from build123d import *

# Parameters (mm, degrees)
F1_DEPTH = 10
F2_R     = 2
F3_R     = 4.4
F4_R     = 4
F5_R     = 6.2


with BuildPart() as f1:
    # F0 (on Top) → F1 (new body)
    with BuildSketch(Plane.XY):
        Polygon((6.78689, 27.703254), (6.78689, 2.703254), (9.18689, 2.703254), (9.18689, 30.103254), (-16.61311, 30.103254), (-16.61311, -19.896746), (-24.81311, -19.896746), (-24.81311, -7.296746), (-27.21311, -7.296746), (-27.21311, -22.296746), (-14.21311, -22.296746), (-14.21311, 27.703254), align=None)
    extrude(amount=F1_DEPTH)

    # F2
    f2_edges = [f1.edges().sort_by_distance(p)[0] for p in [
        (-14.21311, 27.703254, 5),
        (6.78689, 27.703254, 5),
    ]]
    fillet(f2_edges, radius=F2_R)

    # F3
    f3_edges = [f1.edges().sort_by_distance(p)[0] for p in [
        (-16.61311, 30.103254, 5),
        (9.18689, 30.103254, 5),
    ]]
    fillet(f3_edges, radius=F3_R)

    # F4
    f4_edges = [f1.edges().sort_by_distance(p)[0] for p in [
        (-24.81311, -19.896746, 5),
        (-16.61311, -19.896746, 5),
    ]]
    fillet(f4_edges, radius=F4_R)

    # F5
    f5_edges = [f1.edges().sort_by_distance(p)[0] for p in [
        (-27.21311, -22.296746, 5),
        (-14.21311, -22.296746, 5),
    ]]
    fillet(f5_edges, radius=F5_R)


solid = f1.part
Build history of the part. All positions in model axes, mm. A direction names the side the tool comes from. Round coordinates to 2 decimals unless told otherwise and drop trailing zeros. Loops run counter-clockwise (first coordinate to the right, second up) from the corner with the lowest first, then second, coordinate; pieces in that order, holes last. Notation, with made-up numbers: (10.25, -8) -> (44.25, -8) arc R20 ccw to (44.25, 7) -> close; hole circle Ø7 at (44.25, -12.5). An arc over 180 degrees is marked (long way). Use CSV: the item, a comma, the result in double quotes. Start each with the question number.
Q1. Saw through at D-D on y = 0. Give the cut face in (x, z), and give its area (3 significant figures).
Q2. Saw through at B-B on z = 4.5. Give the cut face in (x, y).
Q3. Saw through at A-A on y = 24.5. Give the cut face in (x, z), and give its area (3 significant figures).
Q4. Mould opens along X. For faces 4 (the face through (9.187, 14, 5)), 5 (the face through (-14.213, 5, 5)), 6 (the face through (-26, -7.297, 5)) say: +X half, -X half, draft (parallel to the pull), parting line (faces both ways), or undercut.
Q5. Saw through at C-C on x = -4.5. Give the cut face in (y, z), and give its area (3 significant figures).
Q6. Flat gauge pins, fed straight in: pin 1 Ø2.5 at (y, z) = (-13, 6.5) entering from +X; pin 2 Ø2.5 at (x, z) = (-26.5, 4.5) entering from +Y; pin 3 Ø3 at (y, z) = (-2.5, 6) entering from -X; pin 4 Ø1.5 at (x, y) = (-12.5, -3.5) entering from -Z. Where does each tip first touch, or does it go through?
Q7. Drill centre lines: L1, parallel to X at y = 21, z = 4; L2, parallel to X at y = -15, z = 8.75; L3, parallel to Y at x = -5.5, z = 1. Where is each one in solid material? Low to high.
Q8. Which spindle directions (+Z, -Z, +X, -X, +Y, -Y) get a long thin tool onto all of the face, cutting with end or side? Do faces 1 (the face through (-24.813, -12, 5)), 2 (the face through (-13.643, 27.102, 5.07)), 3 (the face through (8, 2.703, 5)). Say none if no direction does.
Solutions:
1,outline,"(-16.61, 0) -> (-14.21, 0) -> (-14.21, 10) -> (-16.61, 10) -> close"
1,area,"24.0 mm^2"
2,outline,"(-27.21, -16.1) arc R6.2 ccw to (-21.01, -22.3) -> (-20.41, -22.3) arc R6.2 ccw to (-14.21, -16.1) -> (-14.21, 25.7) arc R2 cw to (-12.21, 27.7) -> (4.79, 27.7) arc R2 cw to (6.79, 25.7) -> (6.79, 2.7) -> (9.19, 2.7) -> (9.19, 25.7) arc R4.4 ccw to (4.79, 30.1) -> (-12.21, 30.1) arc R4.4 ccw to (-16.61, 25.7) -> (-16.61, -15.9) arc R4 cw to (-20.61, -19.9) -> (-20.81, -19.9) arc R4 cw to (-24.81, -15.9) -> (-24.81, -7.3) -> (-27.21, -7.3) -> close"
3,outline,"(-16.61, 0) -> (-14.21, 0) -> (-14.21, 10) -> (-16.61, 10) -> close; (6.79, 0) -> (9.19, 0) -> (9.19, 10) -> (6.79, 10) -> close"
3,area,"48.0 mm^2"
4,face 4,"+X half"
4,face 5,"undercut"
4,face 6,"draft"
5,outline,"(27.7, 0) -> (30.1, 0) -> (30.1, 10) -> (27.7, 10) -> close"
5,area,"24.0 mm^2"
6,pin 1,"stops at x = -14.21"
6,pin 2,"stops at y = -7.3"
6,pin 3,"stops at x = -16.61"
6,pin 4,"passes through"
7,L1,"x = -16.61 to -14.21, 6.79 to 9.19"
7,L2,"x = -27.21 to -24.81, -16.61 to -14.21"
7,L3,"y = 27.7 to 30.1"
8,face 1,"+Z, -Z, +Y"
8,face 2,"+Z, -Z, -Y"
8,face 3,"+Z, -Z, +X, -Y"
